Design review of the part built by this model. Coordinates are the model's own, in mm. Coordinates: 2 decimals unless noted, no trailing zeros. Order: outer loops, then holes, each group sorted by start corner. A loop starts at its lowest first (then second) coordinate and runs counter-clockwise, first axis right, second up. Notation, with made-up numbers: (31, 75) -> (45, 75) arc R28 cw to (45, 108) -> close; hole circle Ø10 at (-33, -13). An arc over 180 degrees is marked (long way). Write item = value, one per line.
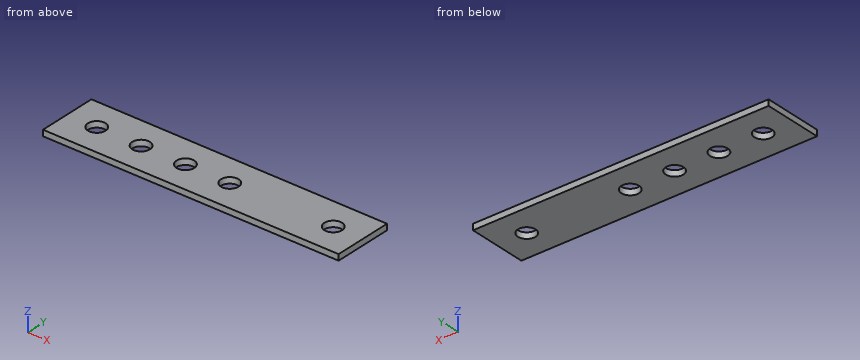
```python
from build123d import *

# Parameters (mm, degrees)
SKETCH1_W           = 200
SKETCH1_H           = 40
SKETCH1_R           = 6
BOSS_EXTRUDE1_DEPTH = 2
SKETCH2_R           = 6
CUT_EXTRUDE1_DEPTH  = 5
LPATTERN1_COUNT     = 4
LPATTERN1_PITCH     = 30


with BuildPart() as part:
    # Sketch1 → Boss-Extrude1 (new body, symmetric)
    with BuildSketch(Plane.XY):
        Rectangle(SKETCH1_W, SKETCH1_H)
        with Locations((80, 0)):
            Circle(SKETCH1_R, mode=Mode.SUBTRACT)
    extrude(amount=BOSS_EXTRUDE1_DEPTH, both=True)

    # Sketch2 → Cut-Extrude1 (cut, through all)
    with BuildSketch(Plane.XY.offset(2)):
        with Locations((-80, 0)):
            Circle(SKETCH2_R)
    cut_extrude1 = extrude(amount=-CUT_EXTRUDE1_DEPTH, mode=Mode.SUBTRACT)

    # LPattern1: Cut-Extrude1 ×4
    with Locations(*[(i * LPATTERN1_PITCH, 0, 0) for i in range(1, LPATTERN1_COUNT)]):
        add(cut_extrude1, mode=Mode.SUBTRACT)


solid = part.part
```
(1) For L1, parallel to X at y = -1, z = 0.7; L2, parallel to Y at x = 10, z = 1.15; L3, parallel to X at y = 4, z = -1.3, list the stretches that pass through material, from the lowest coordinate up.
Report:
L1 = -100 to -85.92, -74.08 to -55.92, -44.08 to -25.92, -14.08 to 4.08, 15.92 to 74.08, 85.92 to 100
L2 = -20 to -6, 6 to 20
L3 = -100 to -84.47, -75.53 to -54.47, -45.53 to -24.47, -15.53 to 5.53, 14.47 to 75.53, 84.47 to 100
(2) Insertion check: pin 1 (11 mm diameter, centred on x = 80, y = 0, fed in from -Z); pin 2 (2 mm diameter, centred on x = -44.5, y = -1.5, fed in from +Z). Each pin has a flat end and moves straight along its axis. Give the tip position at first contact, or say it passes through.
Report:
pin_1 = through
pin_2 = 2
(3) We need section A-A (x = -80). Write out the cut boundary in (y, z).
Report:
outline = (-20, -2) -> (-6, -2) -> (-6, 2) -> (-20, 2) -> close; (6, -2) -> (20, -2) -> (20, 2) -> (6, 2) -> close
(4) We need section B-B (y = 0). Write out the cut boundary in (x, z), and give its area (3 significant figures).
Report:
outline = (-100, -2) -> (-86, -2) -> (-86, 2) -> (-100, 2) -> close; (-74, -2) -> (-56, -2) -> (-56, 2) -> (-74, 2) -> close; (-44, -2) -> (-26, -2) -> (-26, 2) -> (-44, 2) -> close; (-14, -2) -> (4, -2) -> (4, 2) -> (-14, 2) -> close; (16, -2) -> (74, -2) -> (74, 2) -> (16, 2) -> close; (86, -2) -> (100, -2) -> (100, 2) -> (86, 2) -> close
area = 560 mm²
(5) We need section C-C (z = 0.65). Write out the cut boundary in (x, y), and give its area (3 significant figures).
Report:
outline = (-100, -20) -> (100, -20) -> (100, 20) -> (-100, 20) -> close; hole circle Ø12 at (-80, 0); hole circle Ø12 at (-50, 0); hole circle Ø12 at (-20, 0); hole circle Ø12 at (10, 0); hole circle Ø12 at (80, 0)
area = 7,430 mm²
